from build123d import *

# Parameters (mm, degrees)
F0_R     = 2
F0_R_2   = 17.5
F0_R_3   = 1.5
F1_DEPTH = 3
F2_R     = 10
F3_R     = 5


with BuildPart() as f1:
    # F0 (on Top) → F1 (new body)
    with BuildSketch(Plane.XY):
        Polygon((180, 110), (0, 110), (0, 0), (110, 0), (110, 30), (180, 30), align=None)
        with Locations((6, 6)):
            Circle(F0_R, mode=Mode.SUBTRACT)
        with Locations((35, 35)):
            Circle(F0_R_2, mode=Mode.SUBTRACT)
        with Locations((104, 6)):
            Circle(F0_R, mode=Mode.SUBTRACT)
        with Locations((6, 104)):
            Circle(F0_R, mode=Mode.SUBTRACT)
        with Locations((155, 107)):
            Circle(F0_R_3, mode=Mode.SUBTRACT)
    extrude(amount=F1_DEPTH)

    # F2
    f2_edges = [f1.edges().sort_by_distance(p)[0] for p in [
        (110, 30, 1.5),
        (180, 30, 1.5),
        (180, 110, 1.5),
    ]]
    fillet(f2_edges, radius=F2_R)

    # F3
    f3_edges = [f1.edges().sort_by_distance(p)[0] for p in [
        (110, 0, 1.5),
        (0, 0, 1.5),
        (0, 110, 1.5),
    ]]
    fillet(f3_edges, radius=F3_R)


solid = f1.part
Here's how the part is built. I have some questions about the finished solid (model axes, mm). Coordinates: 2 decimals unless noted, no trailing zeros. Write each loop counter-clockwise with the first axis right and the second up, starting at its lowest first coordinate (ties: lowest second). Pieces come first, ordered by that corner, then holes.
Item 1: Will these pins go through, and if not, where does the flat tip stop? pin 1 (1.8 mm diameter, centred on x = 155, y = 107, fed in from +Z) (3 decimals); pin 2 (0.9 mm diameter, centred on x = 137.5, z = 1.5, fed in from -Y).
Item 2: If we mould it in two halves opening along X, with no side actions, what happens to faces 1 (the cylindrical face through (102.526, 7.352, 1.479)), 2 (the cylindrical face through (2, 109, 2)), 3 (the cylindrical face through (177.15, 33.01, 1.52)), 4 (the flat face through (89, 56, 0))? For each: +X half, -X half, draft (parallel to the pull), parting line (faces both ways), or undercut.
Item 3: I want a section at A-A on z = 1.1. Write out the boundary of the cut face in (x, y), and give its area (3 significant figures).
Item 4: If I drill on line 1 (Y direction, x = 6, z = 0.8); line 2 (Y direction, x = 155, z = 1.4); line 3 (Y direction, x = 34, z = 0.3), over which ranges is the centre line in solid material (lowest first)?
Item 5: I want a section at B-B on x = 168. Write out the boundary of the cut face in (y, z), and give its area (3 significant figures).
Findings below:
1. pin 1: passes through
1. pin 2: stops at y = 30
2. face 1: undercut
2. face 2: -X half
2. face 3: +X half
2. face 4: draft
3. outline: (0, 5) arc R5 ccw to (5, 0) - (105, 0) arc R5 ccw to (110, 5) - (110, 20) arc R10 cw to (120, 30) - (170, 30) arc R10 ccw to (180, 40) - (180, 100) arc R10 ccw to (170, 110) - (5, 110) arc R5 ccw to (0, 105) - close; hole circle Ø4 at (6, 6); hole circle Ø4 at (6, 104); hole circle Ø35 at (35, 35); hole circle Ø4 at (104, 6); hole circle Ø3 at (155, 107)
3. area: 16,700 mm2
4. line 1: y = 0 to 4, 8 to 102, 106 to 110
4. line 2: y = 30 to 105.5, 108.5 to 110
4. line 3: y = 0 to 17.53, 52.47 to 110
5. outline: (30, 0) - (110, 0) - (110, 3) - (30, 3) - close
5. area: 240 mm2
